Read the model definition and answer for the solid it produces. Units are mm, in the model's axes. Round coordinates to 2 decimals unless told otherwise and drop trailing zeros. Order: outer loops, then holes, each group sorted by start corner. A loop starts at its lowest first (then second) coordinate and runs counter-clockwise, first axis right, second up. Notation, with made-up numbers: (77.5, 68) -> (104.5, 68) arc R6 cw to (104.5, 74) -> close; hole circle Ø1 at (68, -38). An arc over 180 degrees is marked (long way). Answer as a JSON object with one key per item and string values. Group by question number.
Item 1: Section D-D, the plane x = -1.1 is taken. Write down the section's boundary in (y, z) (3 decimals).
Item 2: The mould has two halves that part along Z. Classify faces 1 (the flat face through (0, 1, -10.16)), 2 (the flat face through (0, 0, -3)), 3 (the flat face through (0, -1.5, 1)), 4 (the flat face through (0, 1.5, -3)): pulls with the +Z half, pulls with the -Z half, needs draft (parallel to the pull), parting line crosses it, or undercut.
Item 3: Section B-B, the plane z = -9 is taken. Write down the section's boundary in (x, y), plus the area to 3 significant figures.
Item 4: Section A-A, the plane x = 0.95 is taken. Write down the section's boundary in (y, z) (3 decimals).
Item 5: Given P1, Ø0.6, axis at x = 0, y = -0.5, coming from the -Z side; P2, Ø0.8, axis at y = -1, z = -1, coming from the +X side; P3, Ø0.8, axis at x = 0, y = -0.5, coming from the +Z side, each flat-ended and moving along its own axis, determine where each tip first touches the part or whether it passes through.
Item 6: Section C-C, the plane y = 2.5 is taken. Count the separate pieces of the cut face and the enclosed holes in it, plus the area to 3 significant figures.
Item 7: Consider probe 1 along Z at (x, y) = (0.25, -0.25); probe 2 along Y at (x, z) = (0.55, -8.5); probe 3 along X at (y, z) = (3, -6.25). Determine where each line is inside the solid, lowest interval first. Write a range as from..to.
from build123d import *

# Parameters (mm, degrees)
BOSS_EXTRUDE1_DEPTH      = 1.5
BOSS_EXTRUDE2_DEPTH      = 6
BOSS_EXTRUDE2_DEPTH_BACK = 3


with BuildPart() as part:
    # Sketch1 → Boss-Extrude1 (new body)
    with BuildSketch(Plane(origin=(0, 0, 0), x_dir=(1, 0, 0), z_dir=(0, 1, 0))):
        Polygon((-0.635, 10.16), (0.635, 10.16), (1.27, 9.525), (1.27, 8.255), (0.635, 7.62), (1.27, 6.985), (1.27, 5.715), (0.635, 5.08), (1.27, 4.445), (1.27, 3.175), (0.635, 2.54), (1.27, 1.905), (1.27, 0.635), (0.635, 0), (1.27, -0.635), (1.27, -1.905), (0.635, -2.54), (1.27, -3.175), (1.27, -4.445), (0.635, -5.08), (-0.635, -5.08), (-1.27, -4.445), (-1.27, -3.175), (-0.635, -2.54), (-1.27, -1.905), (-1.27, -0.635), (-0.635, 0), (-1.27, 0.635), (-1.27, 1.905), (-0.635, 2.54), (-1.27, 3.175), (-1.27, 4.445), (-0.635, 5.08), (-1.27, 5.715), (-1.27, 6.985), (-0.635, 7.62), (-1.27, 8.255), (-1.27, 9.525), align=None)
    extrude(amount=BOSS_EXTRUDE1_DEPTH)

    # Sketch3 → Boss-Extrude2 (add, two sides: drawn at the far end of the back side and taken through both)
    with BuildSketch(Plane(origin=(0, 1.5, 0), x_dir=(1, 0, 0), z_dir=(0, 1, 0)).offset(-BOSS_EXTRUDE2_DEPTH_BACK)):
        Polygon((0.375, 9.39), (0.5, 9.265), (0.5, 8.515), (0.375, 8.39), (-0.375, 8.39), (-0.5, 8.515), (-0.5, 9.265), (-0.375, 9.39), align=None)
        Polygon((0.375, 6.85), (0.5, 6.725), (0.5, 5.975), (0.375, 5.85), (-0.375, 5.85), (-0.5, 5.975), (-0.5, 6.725), (-0.375, 6.85), align=None)
        Polygon((0.375, 4.31), (0.5, 4.185), (0.5, 3.435), (0.375, 3.31), (-0.375, 3.31), (-0.5, 3.435), (-0.5, 4.185), (-0.375, 4.31), align=None)
        Polygon((0.375, 1.77), (0.5, 1.645), (0.5, 0.895), (0.375, 0.77), (-0.375, 0.77), (-0.5, 0.895), (-0.5, 1.645), (-0.375, 1.77), align=None)
        Polygon((0.375, -0.77), (0.5, -0.895), (0.5, -1.645), (0.375, -1.77), (-0.375, -1.77), (-0.5, -1.645), (-0.5, -0.895), (-0.375, -0.77), align=None)
        Polygon((0.375, -3.31), (0.5, -3.435), (0.5, -4.185), (0.375, -4.31), (-0.375, -4.31), (-0.5, -4.185), (-0.5, -3.435), (-0.375, -3.31), align=None)
    extrude(amount=BOSS_EXTRUDE2_DEPTH + BOSS_EXTRUDE2_DEPTH_BACK)


solid = part.part
Values found:
{
 "1": {"outline": "(0, -9.695) -> (1.5, -9.695) -> (1.5, -8.085) -> (0, -8.085) -> close; (0, -7.155) -> (1.5, -7.155) -> (1.5, -5.545) -> (0, -5.545) -> close; (0, -4.615) -> (1.5, -4.615) -> (1.5, -3.005) -> (0, -3.005) -> close; (0, -2.075) -> (1.5, -2.075) -> (1.5, -0.465) -> (0, -0.465) -> close; (0, 0.465) -> (1.5, 0.465) -> (1.5, 2.075) -> (0, 2.075) -> close; (0, 3.005) -> (1.5, 3.005) -> (1.5, 4.615) -> (0, 4.615) -> close"},
 "2": {"face 1": "pulls with the -Z half", "face 2": "undercut", "face 3": "needs draft", "face 4": "undercut"},
 "3": {"outline": "(-1.27, 0) -> (-0.5, 0) -> (-0.5, -1.5) -> (0.5, -1.5) -> (0.5, 0) -> (1.27, 0) -> (1.27, 1.5) -> (0.5, 1.5) -> (0.5, 7.5) -> (-0.5, 7.5) -> (-0.5, 1.5) -> (-1.27, 1.5) -> close", "area": "11.3 mm2"},
 "4": {"outline": "(0, -9.845) -> (1.5, -9.845) -> (1.5, -7.935) -> (0, -7.935) -> close; (0, -7.305) -> (1.5, -7.305) -> (1.5, -5.395) -> (0, -5.395) -> close; (0, -4.765) -> (1.5, -4.765) -> (1.5, -2.855) -> (0, -2.855) -> close; (0, -2.225) -> (1.5, -2.225) -> (1.5, -0.315) -> (0, -0.315) -> close; (0, 0.315) -> (1.5, 0.315) -> (1.5, 2.225) -> (0, 2.225) -> close; (0, 2.855) -> (1.5, 2.855) -> (1.5, 4.765) -> (0, 4.765) -> close"},
 "5": {"P1": "z = -9.39", "P2": "x = 0.5", "P3": "z = 4.31"},
 "6": {"separate pieces": "6", "enclosed holes": "0", "area": "5.81 mm2"},
 "7": {"probe 1": "-9.39..-8.39, -6.85..-5.85, -4.31..-3.31, -1.77..-0.77, 0.77..1.77, 3.31..4.31", "probe 2": "0..1.5", "probe 3": "-0.5..0.5"}
}
